Design review of the part built by this model. Coordinates are the model's own, in mm. A direction names the side the tool comes from. Round coordinates to 2 decimals unless told otherwise and drop trailing zeros. Order: outer loops, then holes, each group sorted by start corner. A loop starts at its lowest first (then second) coordinate and runs counter-clockwise, first axis right, second up. Notation, with made-up numbers: (44, -7.75) - (68, -7.75) arc R23 ccw to (68, 29.25) - close; hole circle Ø4 at (5.5, 43.25). An arc over 180 degrees is marked (long way). Write item = value, one per line.
from build123d import *

# Parameters (mm, degrees)
BOSS_EXTRUDE1_DEPTH = 35
SKETCH2_R           = 11
BOSS_EXTRUDE2_DEPTH = 4
FILLET1_R           = 2.54
FILLET2_R           = 2.54


with BuildPart() as part:
    # Sketch1 → Boss-Extrude1 (new body)
    with BuildSketch(Plane(origin=(0, 0, 0), x_dir=(1, 0, 0), z_dir=(0, 1, 0))):
        with BuildLine():
            Line((-19, -13), (24, -13))
            Line((24, -13), (24, 13))
            Line((24, 13), (-19, 13))
            ThreePointArc((-19, 13), (-22.535533906, 11.535533906), (-24, 8))
            Line((-24, 8), (-24, -8))
            ThreePointArc((-24, -8), (-22.535533906, -11.535533906), (-19, -13))
        make_face()
    extrude(amount=BOSS_EXTRUDE1_DEPTH)

    # Sketch2 → Boss-Extrude2 (add)
    with BuildSketch(Plane(origin=(0, 35, 0), x_dir=(1, 0, 0), z_dir=(0, 1, 0))):
        with Locations(Location((-9.4, 0, 0), (0, 0, 90))):
            Circle(SKETCH2_R)
    extrude(amount=BOSS_EXTRUDE2_DEPTH)

    # Fillet1
    fillet1_edges = [part.edges().sort_by_distance(p)[0] for p in [
        (2.5, 35, 13),
        (-22.535533906, 35, 11.535533906),
        (-24, 35, 0),
        (-22.535533906, 35, -11.535533906),
        (-24, 0, 0),
        (-22.535533906, 0, 11.535533906),
        (2.5, 0, 13),
        (2.5, 35, -13),
        (2.5, 0, -13),
        (-22.535533906, 0, -11.535533906),
    ]]
    fillet(fillet1_edges, radius=FILLET1_R)

    # Fillet2
    fillet2_edges = [part.edges().sort_by_distance(p)[0] for p in [
        (24, 17.5, 13),
        (24, 0, 0),
        (24, 17.5, -13),
        (24, 35, 0),
        (24, 34.256051224, 12.256051224),
        (24, 34.256051224, -12.256051224),
        (24, 0.743948776, -12.256051224),
        (24, 0.743948776, 12.256051224),
    ]]
    fillet(fillet2_edges, radius=FILLET2_R)


solid = part.part
Item 1: Take a section at A-A, the plane x = 7. State the section outline as (y, z) points, and give its area (3 significant figures).
Data:
outline = (0, -10.46) arc R2.54 ccw to (2.54, -13) - (32.46, -13) arc R2.54 ccw to (35, -10.46) - (35, 10.46) arc R2.54 ccw to (32.46, 13) - (2.54, 13) arc R2.54 ccw to (0, 10.46) - close
area = 904 mm2
Item 2: Take a section at C-C, the plane x = -0.5. State the section outline as (y, z) points, and give its area (3 significant figures).
Data:
outline = (0, -10.46) arc R2.54 ccw to (2.54, -13) - (32.46, -13) arc R2.54 ccw to (35, -10.46) - (35, -6.46) - (39, -6.46) - (39, 6.46) - (35, 6.46) - (35, 10.46) arc R2.54 ccw to (32.46, 13) - (2.54, 13) arc R2.54 ccw to (0, 10.46) - close
area = 956 mm2
Item 3: Insertion check: P1, Ø6, axis at x = 14.5, z = 5, coming from the +Y side. The pin has a flat end and moves straight along its axis. Give the tip position at first contact, or say it passes through.
Data:
P1 = 35
Item 4: For faces 1 (the face through (7.924, 34.236, 12.276)), 2 (the face through (-15.859, 34.236, 12.276)), 3 (the face through (7.54, 34.236, -12.276)), 4 (the face through (-15.945, 34.236, -12.276)), list the 3-axis set-ups (+Z, -Z, +X, -X, +Y, -Y) from which the entire face can be reached by the end or side of a thin tool; tool diameter is ignored.
Data:
face_1 = +Z, +X, +Y
face_2 = +Z, -X, +Y
face_3 = -Z, +X, +Y
face_4 = -Z, -X, +Y
Item 5: Take a section at B-B, the plane z = 0. State the section outline as (x, y) points.
Data:
outline = (-24, 2.54) arc R2.54 ccw to (-21.46, 0) - (21.46, 0) arc R2.54 ccw to (24, 2.54) - (24, 32.46) arc R2.54 ccw to (21.46, 35) - (1.6, 35) - (1.6, 39) - (-20.4, 39) - (-20.4, 35) - (-21.46, 35) arc R2.54 ccw to (-24, 32.46) - close
Item 6: For line 1 along Y through (x, z) = (12.5, 2.75); line 2 along X through (y, z) = (33, -3.25); line 3 along X through (y, z) = (2, -11.25), list the stretches that pass through material, from the lowest coordinate up. Write a range as [from, to].
Data:
line_1 = [0, 35]
line_2 = [-23.94, 23.94]
line_3 = [-22.72, 23.81]
